```python
from build123d import *

# Parameters (mm, degrees)
SKETCH_2_W          = 7
SKETCH_2_H          = 7
CUT_EXTRUDE_1_DEPTH = 20
CUT_EXTRUDE_2_DEPTH = 3


with BuildPart() as part:
    # 草图1 → 旋转1 (revolve)
    with BuildSketch(Plane.XY):
        Polygon((0, 0), (-5.5, 0), (-5.5, 50), (-9, 50), (-9, 80), (0, 80), align=None)
    revolve(axis=Axis((0, 0, 0), (0, 1, 0)))

    # 草图2 → 切除-拉伸1 (cut)
    with BuildSketch(Plane(origin=(0, 80, 0), x_dir=(1, 0, 0), z_dir=(0, 1, 0))):
        Rectangle(SKETCH_2_W, SKETCH_2_H)
    extrude(amount=-CUT_EXTRUDE_1_DEPTH, mode=Mode.SUBTRACT)

    # 草图4 → 切除-拉伸2 (cut)
    with BuildSketch(Plane.XY.offset(5.5)):
        with BuildLine():
            Line((-2, 10), (-2, 18))
            ThreePointArc((-2, 18), (0, 20), (2, 18))
            Line((2, 18), (2, 10))
            ThreePointArc((2, 10), (0, 8), (-2, 10))
        make_face()
    extrude(amount=-CUT_EXTRUDE_2_DEPTH, mode=Mode.SUBTRACT)


solid = part.part
```
Verification items for the finished model (mm, model axes). A direction names the side the tool comes from. Give positions to 0.01 mm unless a question says otherwise; leave off trailing zeros. Order: outer loops, then holes, each group sorted by start corner. A loop starts at its lowest first (then second) coordinate and runs counter-clockwise, first axis right, second up. Notation, with made-up numbers: M 51.5,30 L 104.5,30 A24 cw 104.5,47 Z; hole C 34,23 d6. An arc over 180 degrees is marked long. Return JSON: item names as keys, results as strings. Group by question number.
1) Access from +Z, -Z, +X, -X, +Y, -Y to the whole of each face (thin tool, end or side, straight path). Record for faces 4 (the face through (-3.5, 70, 0)), 5 (the face through (0, 20, 4)), 6 (the face through (0, 0, 0)).
2) Section check B-B on x = 0. Record the cut outline in (y, z).
3) Scan lines: line 1 (Y direction, x = -7.5, z = 0); line 2 (Y direction, x = -1, z = 1.75); line 3 (Z direction, x = 1.5, y = 67). Record each from-to range of solid material in increasing order.
4) Section check C-C on y = 23. Record the cut outline in (x, z), and give its area (3 significant figures).
5) Section check A-A on z = 0. Record the cut outline in (x, y), and give its area (3 significant figures).
6) Mould release check, pull along X, two halves, no side actions. Record for faces 1 (the face through (-4, 50, -4)), 2 (the face through (0, 60, 0)), 3 (the face through (1.19, 25.35, -5.37)): pulls with the +X half, pulls with the -X half, needs draft (parallel to the pull), parting line crosses it, or undercut.
7) Section check D-D on x = -4.5. Record the cut outline in (y, z).
8) Go/stop test with flat-tipped pins: pin 1 Ø10 at (x, y) = (2, 32.5) entering from -Z; pin 2 Ø3 at (x, y) = (-1, 11.5) entering from +Z; pin 3 Ø6 at (y, z) = (46, -6.5) entering from -X; pin 4 Ø1.5 at (y, z) = (8.5, -6.5) entering from +X. Record where each tip stops, or that it passes through.
Answer block:
{
 "1": {"face 4": "+Y", "face 5": "+Z", "face 6": "+Z, -Z, +X, -X, -Y"},
 "2": {"outline": "M 0,-5.5 L 50,-5.5 L 50,-9 L 80,-9 L 80,-3.5 L 60,-3.5 L 60,3.5 L 80,3.5 L 80,9 L 50,9 L 50,5.5 L 20,5.5 L 20,2.5 L 8,2.5 L 8,5.5 L 0,5.5 Z"},
 "3": {"line 1": "y = 50 to 80", "line 2": "y = 0 to 60", "line 3": "z = -8.87 to -3.5, 3.5 to 8.87"},
 "4": {"outline": "C 0,0 d11", "area": "95.0 mm^2"},
 "5": {"outline": "M -9,50 L -5.5,50 L -5.5,0 L 5.5,0 L 5.5,50 L 9,50 L 9,80 L 3.5,80 L 3.5,60 L -3.5,60 L -3.5,80 L -9,80 Z", "area": "950 mm^2"},
 "6": {"face 1": "needs draft", "face 2": "undercut", "face 3": "parting line crosses it"},
 "7": {"outline": "M 0,-3.16 L 50,-3.16 L 50,-7.79 L 80,-7.79 L 80,7.79 L 50,7.79 L 50,3.16 L 0,3.16 Z"},
 "8": {"pin 1": "stops at z = -5.5", "pin 2": "stops at z = 5.12", "pin 3": "stops at x = -4.24", "pin 4": "passes through"}
}
